Autodesk Inventor part; units mm, degrees
ref_plane "YZ Plane" through (0, 0, 0) normal (1, 0, 0) x (0, 1, 0)
ref_plane "XZ Plane" through (0, 0, 0) normal (0, 1, 0) x (-1, 0, 0)
ref_plane "XY Plane" through (0, 0, 0) normal (0, 0, 1) x (1, 0, 0)
sketch "Sketch1" plane through (0, 0, 0) normal (0, 1, 0) x (-1, 0, 0)
  circle A0 centre (0, 0) radius 5
  line L0 (-6, 85) -> (6, 85)
  arc A1 (-6, 3.6056) -> (6, 3.6056) centre (0, 0) ccw
  line L1 (-6, 3.6056) -> (-6, 85)
  line L2 (6, 85) -> (6, 3.6056)
  point P0 (-6, 0)
  point P1 (-5, 85)
  point P2 (5, 85)
extrude "Extrusion1" add sketch "Sketch1" along normal blind 5
sketch "Sketch2" plane through (0, 5, 0) normal (0, 1, 0) x (1, 0, 0)
  line L0 (-6, -85) -> (6, -85) construction
  line L1 (0, -85) -> (0, -75) construction
  point P0 (0, 0)
  point P1 (-5, -85)
  point P2 (5, -85)
  dimension "d5" = 10
hole "Hole1" at (0, 5, 75) direction (0, -1, 0) diameter 5.1 end through all
draft "FaceDraft1" angle 15 pull direction (0, 1, 0) faces at (-4.9353, 3.3333, -0.8021) fixed edges at (5, 5, 0)
sketch "Sketch3" plane through (0, 0, 0) normal (0, -1, 0) x (1, 0, 0)
  line L0 (0, 0) -> (-10, 0)
  line L1 (-10, 0) -> (-10, 0.6)
  line L2 (-10, 0.6) -> (0, 0.6)
  line L3 (0, 0.6) -> (0, 0)
  dimension "d15" = 0.6
  dimension "d19" = 10
extrude "Extrusion2" cut sketch "Sketch3" against normal blind 10
fillet "Fillet2" radius 0.5 2 edges at (-4.2347, 2.3015, 0.6) (-4.3301, 2.5, 0)
sketch "Sketch4" plane through (0, 0, 0) normal (0, -1, 0) x (1, 0, 0)
  line L0 (6, 85) -> (-6, 85) construction
  line L1 (0, 85) -> (0, 65) construction
  line L2 (5, 84) -> (5, 4.3589)
  line L3 (-5, 4.3589) -> (-5, 84)
  line L4 (5, 65) -> (-5, 65)
  line L5 (-5, 65) -> (-5, 63)
  line L6 (-5, 63) -> (5, 63)
  line L7 (5, 63) -> (5, 65)
  line L8 (-5, 77.5) -> (5, 77.5)
  line L9 (5, 77.5) -> (5, 72.5)
  line L10 (5, 72.5) -> (-5, 72.5)
  line L11 (-5, 72.5) -> (-5, 77.5)
  line L12 (-5, 77.5) -> (5, 72.5) construction
  line L13 (5, 77.5) -> (-5, 72.5) construction
  circle A0 centre (0, 75) radius 2.55
  point P0 (0, 0)
  point P1 (4, 85)
  point P2 (-4, 85)
  dimension "d21" = 20
  dimension "d22" = 2
  dimension "d23" = 5
extrude "Extrusion3" add sketch "Sketch4" along normal blind 2 contours L2 L10 A0 L8 | L2 L6 L3 L4 | A0 L10 L3 L8
sketch "Sketch5" plane through (0, -2, 0) normal (0, -1, 0) x (1, 0, 0)
  arc A0 (0.5025, 72.5) -> (0.5025, 77.5) centre (0, 75) ccw
  circle A1 centre (0, 75) radius 2.55
  line L0 (2.55, 77.55) -> (-2.55, 77.55)
  line L1 (-2.55, 77.55) -> (-2.55, 72.45)
  line L2 (-2.55, 72.45) -> (2.55, 72.45)
  line L3 (2.55, 72.45) -> (2.55, 77.55)
  line L4 (2.55, 77.55) -> (-2.55, 72.45) construction
  line L5 (-2.55, 77.55) -> (2.55, 72.45) construction
  arc A2 (-0.5025, 72.5) -> (0.5025, 72.5) centre (0, 75) ccw
  arc A3 (0.5025, 77.5) -> (-0.5025, 77.5) centre (0, 75) ccw
  arc A4 (-0.5025, 77.5) -> (-0.5025, 72.5) centre (0, 75) ccw
  point P0 (0, 0)
  dimension "d26" = 5.1
  dimension "d27" = 5.1
extrude "Extrusion4" cut sketch "Sketch5" against normal blind 2 contours A0 L3 L2 A1 | A0 A1 L0 L3 | L2 L1 A1 | A1 L1 L0
sketch "Sketch6" plane through (-5, 0, 72.5) normal (-1, 0, 0) x (0, 0, 1)
  line L0 (0, 0) -> (5, 0)
  line L1 (0, 0) -> (0, -2)
  line L2 (5, -2) -> (0, -2)
  line L3 (5, 0) -> (5, -2)
  line L4 (-9.5, 0) -> (-7.5, 0)
  line L5 (-9.5, 0) -> (-9.5, -2)
  line L6 (-7.5, -2) -> (-9.5, -2)
  line L7 (-7.5, 0) -> (-7.5, -2)
  point P0 (-72.5, 0)
extrude "Extrusion5" add sketch "Sketch6" along normal blind 1
sketch "Sketch7" plane through (5, 0, 77.5) normal (1, 0, 0) x (0, 0, -1)
  line L0 (0, 0) -> (5, 0)
  line L1 (0, 0) -> (0, -2)
  line L2 (5, -2) -> (0, -2)
  line L3 (5, 0) -> (5, -2)
  line L4 (12.5, 0) -> (14.5, 0)
  line L5 (12.5, 0) -> (12.5, -2)
  line L6 (14.5, -2) -> (12.5, -2)
  line L7 (14.5, 0) -> (14.5, -2)
  point P0 (77.5, 0)
extrude "Extrusion6" add sketch "Sketch7" along normal blind 1
fillet "Fillet4" radius 1 4 edges at (6, 2.5, 85) (-6, 2.5, 85) (6, 2.5, 3.6056) (-6, 2.5, 3.6056)
properties part number "filament guide stronger"
Can you work these out from the model? Positions are in its coordinate system, mm. A direction names the side the tool comes from. Round coordinates to 2 decimals unless told otherwise and drop trailing zeros. Order: outer loops, then holes, each group sorted by start corner. A loop starts at its lowest first (then second) coordinate and runs counter-clockwise, first axis right, second up. Notation, with made-up numbers: (4, 6.5) - (54, 6.5) arc R26 cw to (54, 39.5) - close; hole circle Ø4 at (-22, -6). An arc over 180 degrees is marked (long way). Answer in a Markdown table with one row per item.
(1) Which directions (+Z, -Z, +X, -X, +Y, -Y) give clear straight access to the entire face, cutting with the end or side of a thin tool? Please do faces 4 (the face through (4, -1, 72.5)), 5 (the face through (0, -1, 63)), 6 (the face through (2.55, -1, 75)), 7 (the face through (-6, 2, 0)), 8 (the face through (6, 2, 43)).
From the geometry:
| item | result |
|---|---|
| face 4 | +X, -X, -Y |
| face 5 | -Z, +X, -X, -Y |
| face 6 | +Z, -Y |
| face 7 | -X, +Y, -Y |
| face 8 | +Z, +X, +Y, -Y |
(2) Please list where these lines run through material, in increasing order: L1, parallel to X at y = 3.45, z = 75; L2, parallel to Z at x = 0, y = 3.2; L3, parallel to Z at x = -0.75, y = 1.5. Write a range as from..to.
From the geometry:
| item | result |
|---|---|
| L1 | x = -6..-2.55, 2.55..6 |
| L2 | z = -7..-4.52, 4.52..72.45, 77.55..85 |
| L3 | z = -6.96..-3.99, 3.99..72.56, 77.44..85 |
(3) If we mould it in two halves opening along X, with no side actions, what happens to faces 1 (the face through (-6, 2, 44)), 2 (the face through (-2.55, -1, 75)), 3 (the face through (0, -1, 65))? For each: released by +X, released by -X, zero draft, split by the parting line, or undercut.
From the geometry:
| item | result |
|---|---|
| face 1 | released by -X |
| face 2 | undercut |
| face 3 | zero draft |
(4) Suppose I cut it at A-A, the plane z = 70. Please give me the cut outline in (x, y).
From the geometry:
| item | result |
|---|---|
| outline | (-6, 0) - (6, 0) - (6, 5) - (-6, 5) - close |
(5) For P1, Ø1.6, axis at x = 4.5, y = -1, coming from the -Z side; P2, Ø0.6, axis at x = 4, y = -1.5, coming from the +Z side; P3, Ø1, axis at x = -1, z = 50.5, coming from the -Y side, each with a flat end and sliding along its axis, tell me the tip position at first contact or that it passes through.
From the geometry:
| item | result |
|---|---|
| P1 | stops at z = 63 |
| P2 | stops at z = 77.5 |
| P3 | stops at y = 0 |
